Autodesk Inventor part; units mm, degrees
ref_plane "YZ Plane" through (0, 0, 0) normal (1, 0, 0) x (0, 1, 0)
ref_plane "XZ Plane" through (0, 0, 0) normal (0, 1, 0) x (-1, 0, 0)
ref_plane "XY Plane" through (0, 0, 0) normal (0, 0, 1) x (1, 0, 0)
sketch "Sketch1" plane through (0, 0, 0) normal (0, 1, 0) x (-1, 0, 0)
  line L0 (0, 0) -> (66, 0)
  line L1 (66, 0) -> (66, -100)
  line L2 (66, -100) -> (0, -100)
  line L3 (0, -100) -> (0, 0)
  line L4 (66, 0) -> (54, 0)
  line L5 (54, 0) -> (54, -12)
  line L6 (54, -12) -> (66, -12)
  line L7 (66, -12) -> (66, 0)
  line L8 (0, 0) -> (12, 0)
  line L9 (12, 0) -> (12, -12)
  line L10 (12, -12) -> (0, -12)
  line L11 (0, -12) -> (0, 0)
  line L12 (0, -100) -> (12, -100)
  line L13 (12, -100) -> (12, -88)
  line L14 (12, -88) -> (0, -88)
  line L15 (0, -88) -> (0, -100)
  line L16 (66, -100) -> (54, -100)
  line L17 (54, -100) -> (54, -88)
  line L18 (54, -88) -> (66, -88)
  line L19 (66, -88) -> (66, -100)
  dimension "d0" = 66
  dimension "d1" = 100
  dimension "d2" = 12
  dimension "d3" = 12
  dimension "d4" = 12
  dimension "d5" = 12
  dimension "d6" = 12
  dimension "d7" = 12
  dimension "d8" = 12
  dimension "d9" = 12
extrude "Extrusion1" add sketch "Sketch1" along normal blind 12 contours L0 L5 L6 L1 L18 L17 L2 L13 L14 L3 L10 L9
sketch "Sketch5" plane through (-66, 0, -88) normal (-1, 0, 0) x (0, 0, 1)
  line L0 (0, 12) -> (-12, 12)
  line L1 (0, 12) -> (12, 12)
  line L2 (12, 12) -> (12, 0)
  line L3 (12, 0) -> (0, 0)
  line L4 (0, 0) -> (0, 12)
  line L5 (76, 12) -> (64, 12)
  line L6 (64, 12) -> (64, 0)
  line L7 (64, 0) -> (76, 0)
  line L8 (76, 0) -> (76, 12)
  point P0 (88, 0)
  dimension "d42" = 12
  dimension "d43" = 12
  dimension "d44" = 12
  dimension "d45" = 12
  dimension "d46" = 12
extrude "Extrusion5" cut sketch "Sketch5" against normal blind 12
sketch "Sketch6" plane through (0, 0, -12) normal (1, 0, 0) x (0, 0, -1)
  line L0 (76, 0) -> (76, 12)
  line L1 (64, 12) -> (12, 12)
  line L2 (76, 0) -> (64, 0)
  line L3 (64, 0) -> (64, 12)
  line L4 (64, 12) -> (76, 12)
  line L5 (76, 12) -> (76, 0)
  line L6 (64, 0) -> (12, 0)
  line L7 (12, 12) -> (-12, 12)
  line L8 (0, 0) -> (12, 0)
  line L9 (12, 0) -> (12, 12)
  line L10 (12, 12) -> (0, 12)
  line L11 (0, 12) -> (0, 0)
  point P0 (-12, 0)
  dimension "d49" = 12
  dimension "d50" = 12
extrude "Extrusion6" cut sketch "Sketch6" against normal blind 12 contours L2 L3 L4 L0 | L8 L11 L7 L9
sketch "Sketch7" plane through (-12, -12, -100) normal (1, 0, 0) x (0, 0, -1)
  circle A0 centre (-18, 18) radius 3
  circle A1 centre (-82, 18) radius 3
  line L0 (-100, 24) -> (-76, 24)
  line L1 (-76, 24) -> (-76, 12)
  line L2 (-24, 12) -> (-24, 24)
  line L3 (-24, 24) -> (0, 24)
  point P0 (-100, 12)
  dimension "d53" = 6
  dimension "d54" = 6
  dimension "d55" = 6
  dimension "d56" = 6
  dimension "d57" = 6
  dimension "d58" = 6
extrude "Extrusion7" cut sketch "Sketch7" against normal up to next
sketch "Sketch8" plane through (0, 0, 0) normal (0, -1, 0) x (1, 0, 0)
  circle A0 centre (-20, -6) radius 3.5
  circle A1 centre (-39, -6) radius 3.5
  circle A2 centre (-20, -94) radius 3.5
  circle A3 centre (-39, -94) radius 3.5
  line L0 (-12, -100) -> (-54, -100)
  line L1 (-54, 0) -> (-12, 0)
  line L2 (-12, 0) -> (-12, -24)
  line L3 (-12, -100) -> (-12, -76)
  point P0 (0, 0)
  dimension "d61" = 7
  dimension "d62" = 7
  dimension "d63" = 7
  dimension "d64" = 6
  dimension "d65" = 7
  dimension "d66" = 6
  dimension "d67" = 6
  dimension "d68" = 6
  dimension "d69" = 8
  dimension "d70" = 19
  dimension "d71" = 8
  dimension "d72" = 19
extrude "Extrusion8" cut sketch "Sketch8" against normal blind 6
properties part number "frameBack"
CAD build for the part. Positions are in the model's coordinates, mm. A direction names the side the tool comes from. Give positions to 0.01 mm unless a question says otherwise; leave off trailing zeros. Loops run counter-clockwise (first coordinate to the right, second up) from the corner with the lowest first, then second, coordinate; pieces in that order, holes last. Notation, with made-up numbers: (67.5, -18.75) - (110.5, -18.75) arc R26 ccw to (110.5, 5.25) - close; hole circle Ø10 at (26, 40.25). An arc over 180 degrees is marked (long way). Put each result on its own line as item: value.
Q1. Slice it at B-B (y = 1.25). Give the cut face in (x, z).
Filled in:
outline: (-66, -76) - (-54, -76) - (-54, -100) - (-12, -100) - (-12, -76) - (0, -76) - (0, -24) - (-12, -24) - (-12, 0) - (-54, 0) - (-54, -24) - (-66, -24) - close; hole circle Ø7 at (-39, -94); hole circle Ø7 at (-39, -6); hole circle Ø7 at (-20, -94); hole circle Ø7 at (-20, -6)
Q2. Mould opens along Y. For faces 5 (the face through (-32.7, 4.2, -79.6)), 6 (the face through (-33, 0, -49)), 7 (the face through (-66, 6, -50)) say: pulls with the +Y half, pulls with the -Y half, needs draft (parallel to the pull), parting line crosses it, or undercut.
Filled in:
face 5: undercut
face 6: pulls with the -Y half
face 7: needs draft
Q3. Slice it at A-A (z = -82). Give the cut face in (x, y).
Filled in:
outline: (-54, 0) - (-12, 0) - (-12, 3) - (-54, 3) - close; (-54, 9) - (-12, 9) - (-12, 12) - (-54, 12) - close
Q4. Flat gauge pins, fed straight in: pin 1 (6.5 mm diameter, centred on x = -20, z = -6, fed in from -Y); pin 2 (6 mm diameter, centred on y = 9, z = -93, fed in from +X); pin 3 (7 mm diameter, centred on y = 6, z = -18, fed in from -X); pin 4 (5 mm diameter, centred on y = 6, z = -82, fed in from -X). Where does each tip first touch, or does it go through?
Filled in:
pin 1: stops at y = 6
pin 2: stops at x = -12
pin 3: stops at x = -54
pin 4: passes through
Q5. Slice it at C-C (x = -20). Give the cut face in (y, z), plus the area to 3 significant figures.
Filled in:
outline: (0, -100) - (12, -100) - (12, 0) - (0, 0) - (0, -2.5) - (6, -2.5) - (6, -9.5) - (0, -9.5) - (0, -90.5) - (6, -90.5) - (6, -97.5) - (0, -97.5) - close; hole circle Ø6 at (6, -82); hole circle Ø6 at (6, -18)
area: 1,060 mm²
Q6. Slice it at D-D (z = -6). Give the cut face in (x, y).
Filled in:
outline: (-54, 0) - (-42.5, 0) - (-42.5, 6) - (-35.5, 6) - (-35.5, 0) - (-23.5, 0) - (-23.5, 6) - (-16.5, 6) - (-16.5, 0) - (-12, 0) - (-12, 12) - (-54, 12) - close
Q7. Tool access for faces 1 (the face through (-60, 6, -24)), 2 (the face through (-39, 6, -94)), 3 (the face through (-6, 6, -76)), 4 (the face through (-12, 6, -12)): list every direction of +Z, -Z, +X, -X, +Y, -Y with a clear straight run to the whole face (end or side of a thin tool).
Filled in:
face 1: +Z, -X, +Y, -Y
face 2: -Y
face 3: -Z, +X, +Y, -Y
face 4: +Z, +X, +Y, -Y
Q8. Probe line 1 along Z through (x, y) = (-24, 7.25); line 2 along Z through (x, y) = (-50.5, 4.25); line 3 along Z through (x, y) = (-20, 3.4). List the from-to ranges inside material, lowest first.
Filled in:
line 1: z = -100 to -84.73, -79.27 to -20.73, -15.27 to 0
line 2: z = -100 to -84.44, -79.56 to -20.44, -15.56 to 0
line 3: z = -100 to -97.5, -90.5 to -83.5, -80.5 to -19.5, -16.5 to -9.5, -2.5 to 0
